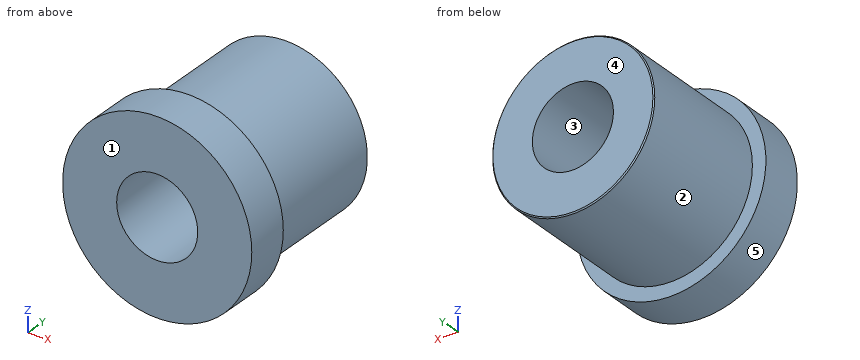
```python
from build123d import *

# Parameters (mm, degrees)
F0_R     = 44.45
F1_DEPTH = 20.32
F2_R     = 38.1
F3_DEPTH = 63.5
F4_SIZE  = 0.508
F6_D     = 38.1


with BuildPart() as f1:
    # F0 (on Front) → F1 (new body)
    with BuildSketch(Plane.XZ):
        Circle(F0_R)
    extrude(amount=F1_DEPTH)

    # F2 (on face) → F3 (join)
    with BuildSketch(Plane(origin=(0, 0, 0), x_dir=(-1, 0, 0), z_dir=(0, 1, 0))):
        Circle(F2_R)
    extrude(amount=F3_DEPTH)

    # F4
    f4_edges = [f1.edges().sort_by_distance(p)[0] for p in [
        (38.1, 63.5, 0),
    ]]
    chamfer(f4_edges, length=F4_SIZE)

    # F6 (through all)
    with Locations(Plane.XZ.offset(20.32)):
        with Locations((0, 0)):
            Hole(F6_D / 2)


solid = f1.part
```
Build history of the part. All positions in model axes, mm. Face numbers are marked on the shaded views. A direction names the side the tool comes from. Round coordinates to 2 decimals unless told otherwise and drop trailing zeros. Order: outer loops, then holes, each group sorted by start corner. A loop starts at its lowest first (then second) coordinate and runs counter-clockwise, first axis right, second up. Notation, with made-up numbers: (72.25, 29.25) - (127.25, 29.25) arc R26 cw to (127.25, 47.25) - close; hole circle Ø7 at (29, 65.25). An arc over 180 degrees is marked (long way). Use a Markdown table: item, result.
1) Wall check: L1, parallel to Z at x = 0, y = 3; L2, parallel to Z at x = 15, y = 8.5; L3, parallel to Y at x = 39, z = -3. Give the ranges that are in metal, low to high.
Recorded:
| item | result |
|---|---|
| L1 | z = -38.1 to -19.05, 19.05 to 38.1 |
| L2 | z = -35.02 to -11.74, 11.74 to 35.02 |
| L3 | y = -20.32 to 0 |
2) Saw through at C-C on y = -14. Write the cut outline in (x, z), and give its area (3 significant figures).
Recorded:
| item | result |
|---|---|
| outline | circle Ø88.9 at (0, 0); hole circle Ø38.1 at (0, 0) |
| area | 5,070 mm² |
3) Flat gauge pins, fed straight in: pin 1 Ø1 at (y, z) = (22, -26.5) entering from +X; pin 2 Ø8 at (x, y) = (-26, -9.5) entering from -Z; pin 3 Ø5 at (y, z) = (54, -21.5) entering from +X. Where does each tip first touch, or does it go through?
Recorded:
| item | result |
|---|---|
| pin 1 | stops at x = 27.85 |
| pin 2 | stops at z = -38.62 |
| pin 3 | stops at x = 33.02 |
4) Saw through at D-D on y = 28. Write the cut outline in (x, z), and give its area (3 significant figures).
Recorded:
| item | result |
|---|---|
| outline | circle Ø76.2 at (0, 0); hole circle Ø38.1 at (0, 0) |
| area | 3,420 mm² |
5) Saw through at A-A on z = 0. Write the cut outline in (x, y), and give its area (3 significant figures).
Recorded:
| item | result |
|---|---|
| outline | (-44.45, -20.32) - (-19.05, -20.32) - (-19.05, 63.5) - (-37.59, 63.5) - (-38.1, 62.99) - (-38.1, 0) - (-44.45, 0) - close; (19.05, -20.32) - (44.45, -20.32) - (44.45, 0) - (38.1, 0) - (38.1, 62.99) - (37.59, 63.5) - (19.05, 63.5) - close |
| area | 3,450 mm² |
6) Tool access for the marked faces 1 and 2: list every direction of +Z, -Z, +X, -X, +Y, -Y with a clear straight run to the whole face (end or side of a thin tool).
Recorded:
| item | result |
|---|---|
| face 1 | +Z, -Z, +X, -X, -Y |
| face 2 | +Y |
7) Saw through at B-B on x = 0. Write the cut outline in (y, z), and give its area (3 significant figures).
Recorded:
| item | result |
|---|---|
| outline | (-20.32, -44.45) - (0, -44.45) - (0, -38.1) - (62.99, -38.1) - (63.5, -37.59) - (63.5, -19.05) - (-20.32, -19.05) - close; (-20.32, 19.05) - (63.5, 19.05) - (63.5, 37.59) - (62.99, 38.1) - (0, 38.1) - (0, 44.45) - (-20.32, 44.45) - close |
| area | 3,450 mm² |
8) Pull direction Z, two halves, no side cores. Call the marked faces 3, 4 and 5: pulls with the +Z half, pulls with the -Z half, needs draft (parallel to the pull), parting line crosses it, or undercut.
Recorded:
| item | result |
|---|---|
| face 3 | undercut |
| face 4 | needs draft |
| face 5 | parting line crosses it |
